Here's how the part is built. I have some questions about the finished solid (model axes, mm). Face numbers are marked on the shaded views. A direction names the side the tool comes from. Give positions to 0.01 mm unless a question says otherwise; leave off trailing zeros. Write each loop counter-clockwise with the first axis right and the second up, starting at its lowest first coordinate (ties: lowest second). Pieces come first, ordered by that corner, then holes. Notation, with made-up numbers: (84, 65) -> (107, 65) arc R12 ccw to (107, 88) -> close; hole circle Ø7 at (61, 83). An arc over 180 degrees is marked (long way). Put each result on its own line as item: value. Start each with the question number.
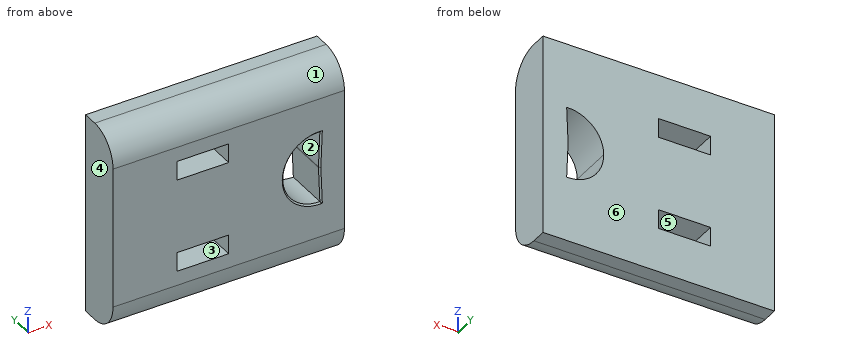
from build123d import *

# Parameters (mm, degrees)
F0_W         = 39.0713959932
F0_H         = 34.1874808073
F0_W_2       = 8.7503567338
F0_H_2       = 3.2559484243
F1_DEPTH     = 7.62
F2_R         = 5.08
F3_R         = 5.08
F4_T2_ANGLE  = 99.0884829953
F4_T4_ANGLE  = 99.0884829953
F4_T8_DEPTH  = 7.3218336241
F4_S9_R      = 6.0154186662
F4_T10_DEPTH = 5
F4_T14_DEPTH = 7.3218336241
F4_S15_R     = 6.0154186662
F4_T16_DEPTH = 5
F4_T21_DEPTH = 7.3218336241
F4_S22_R     = 6.0154186662
F4_T23_DEPTH = 5
F4_T26_ANGLE = 105.3128275547
F4_T33_ANGLE = 105.3128275547
F4_T37_DEPTH = 7.3218336241
F4_S38_R     = 6.0154186662
F4_T39_DEPTH = 5


# Not quite as in the source:
# - a fillet or chamfer that OpenCascade refuses, or shapes differently, is made with other operations: its cross-section is extruded or revolved along the edge and cut away or added


with BuildPart() as f1:
    # F0 (on Front) → F1 (new body)
    with BuildSketch(Plane.XZ):
        with Locations((19.5356979966, 17.0937404037)):
            Rectangle(F0_W, F0_H)
        with Locations((15.1605196297, 9.1573596001)):
            Rectangle(F0_W_2, F0_H_2, mode=Mode.SUBTRACT)
        with Locations((15.1605196297, 25.0301212072)):
            Rectangle(F0_W_2, F0_H_2, mode=Mode.SUBTRACT)
        with BuildLine():
            ThreePointArc((28.8283239088, 17.0937404037), (30.6523842077, 21.4714728973), (35.0814722478, 23.1670308858))
            Line((35.0814722478, 23.1670308858), (34.8434170056, 17.1563244854))
            Line((34.8434170056, 17.1563244854), (34.8434170056, 17.0311563219))
            Line((34.8434170056, 17.0311563219), (35.0814722478, 11.0204499215))
            ThreePointArc((35.0814722478, 11.0204499215), (30.6523842077, 12.71600791), (28.8283239088, 17.0937404037))
        make_face(mode=Mode.SUBTRACT)
    extrude(amount=F1_DEPTH)

    # F2
    f2_edges = [f1.edges().sort_by_distance(p)[0] for p in [
        (19.535698, -7.62, 34.187481),
    ]]
    fillet(f2_edges, radius=F2_R)

    # F3
    f3_edges = [f1.edges().sort_by_distance(p)[0] for p in [
        (19.535698, -7.62, 0),
    ]]
    fillet(f3_edges, radius=F3_R)

    # F4: chamfer of 0.254 on 4 edges, made by hand

    # F4_s1 → F4_t2 (revolve, cut)
    with BuildSketch(Plane(origin=(35.4623142005, 0, 1.4044921235), x_dir=(0, 1, 0), z_dir=(0.9992166354, 0, 0.0395741769))):
        Polygon((-7.62, 9.3694965041), (-7.366, 9.6234965041), (-7.62, 9.6234965041), align=None)
    revolve(axis=Axis((34.8434170056, -7.62, 17.0311563219), (0, 1, 0)), revolution_arc=F4_T2_ANGLE, mode=Mode.SUBTRACT)

    # F4_s3 → F4_t4 (revolve, cut)
    with BuildSketch(Plane(origin=(-1.5316236266, 0, 12.8056905764), x_dir=(0, 1, 0), z_dir=(0.1187584985, 0, -0.9929231688))):
        Polygon((-7.62, 30.3648766921), (-7.366, 30.6188766921), (-7.62, 30.6188766921), align=None)
    revolve(axis=Axis((34.8434170056, -7.62, 17.1563244854), (0, 1, 0)), revolution_arc=F4_T4_ANGLE, mode=Mode.SUBTRACT)


with BuildPart() as f4_tool6:
    # F4_s7 → F4_t8 (new body)
    with BuildSketch(Plane(origin=(0.9968897612, 0, 25.170677246), x_dir=(0, 1, 0), z_dir=(-0.0395741769, 0, -0.9992166354))):
        Polygon((-7.62, 34.3911744878), (-7.366, 34.1371744878), (-7.62, 34.1371744878), align=None)
    extrude(amount=F4_T8_DEPTH)

    # F4_s9 → F4_t10 (intersect, symmetric)
    with BuildSketch(Plane.XZ.offset(7.5)):
        with Locations((34.8434170056, 17.1563244854)):
            Circle(F4_S9_R)
    extrude(amount=F4_T10_DEPTH, both=True, mode=Mode.INTERSECT)


with BuildPart() as f1_1:
    add(f1.part)

    # F4_t5: cut F4_tool6
    add(f4_tool6.part, mode=Mode.SUBTRACT)


with BuildPart() as f4_tool12:
    # F4_s13 → F4_t14 (new body)
    with BuildSketch(Plane(origin=(-0.6447473432, 0, 16.2793599777), x_dir=(0, 1, 0), z_dir=(0.0395741769, 0, -0.9992166354))):
        Polygon((-7.62, 35.7441158998), (-7.366, 35.4901158998), (-7.62, 35.4901158998), align=None)
    extrude(amount=F4_T14_DEPTH)

    # F4_s15 → F4_t16 (intersect, symmetric)
    with BuildSketch(Plane.XZ.offset(7.5)):
        with Locations((34.8434170056, 17.0311563219)):
            Circle(F4_S15_R)
    extrude(amount=F4_T16_DEPTH, both=True, mode=Mode.INTERSECT)


with BuildPart() as f1_2:
    add(f1_1.part)

    # F4_t11: cut F4_tool12
    add(f4_tool12.part, mode=Mode.SUBTRACT)


with BuildPart() as f4_tool19:
    # F4_s20 → F4_t21 (new body)
    with BuildSketch(Plane(origin=(-0.6447473432, 0, 16.2793599777), x_dir=(0, 1, 0), z_dir=(0.0395741769, 0, -0.9992166354))):
        Polygon((-7.62, 35.7441158998), (-7.366, 35.4901158998), (-7.62, 35.4901158998), align=None)
    extrude(amount=F4_T21_DEPTH)

    # F4_s22 → F4_t23 (cut, symmetric)
    with BuildSketch(Plane.XZ.offset(7.5)):
        with Locations((34.8434170056, 17.0311563219)):
            Circle(F4_S22_R)
    extrude(amount=F4_T23_DEPTH, both=True, mode=Mode.SUBTRACT)


with BuildPart() as f4_tool24:
    # F4_s25 → F4_t26 (revolve)
    with BuildSketch(Plane(origin=(36.5710723448, 0, 5.4606046716), x_dir=(0, 1, 0), z_dir=(0.9890355378, 0, 0.1476777062))):
        Polygon((-7.62, 5.4294042858), (-7.366, 5.6834042858), (-7.62, 5.6834042858), align=None)
    revolve(axis=Axis((34.8434170056, -7.62, 17.0311563219), (0, 1, 0)), revolution_arc=F4_T26_ANGLE)

    split(bisect_by=Plane(origin=(35.4623142005, 0, 1.4044921235), x_dir=(0, 1, 0), z_dir=(0.9992166354, 0, 0.0395741769)), keep=Keep.TOP)


with BuildPart() as f4_tool19_1:
    add(f4_tool19.part)

    # F4_t28: intersect F4_tool24
    add(f4_tool24.part, mode=Mode.INTERSECT)


with BuildPart() as f1_3:
    add(f1_2.part)

    # F4_t17: cut F4_tool19
    add(f4_tool19_1.part, mode=Mode.SUBTRACT)


with BuildPart() as f4_tool31:
    # F4_s32 → F4_t33 (revolve)
    with BuildSketch(Plane(origin=(-1.5316236266, 0, 12.8056905764), x_dir=(0, 1, 0), z_dir=(0.1187584985, 0, -0.9929231688))):
        Polygon((-7.62, 30.3648766921), (-7.366, 30.6188766921), (-7.62, 30.6188766921), align=None)
    revolve(axis=Axis((34.8434170056, -7.62, 17.1563244854), (0, 1, 0)), revolution_arc=F4_T33_ANGLE)

    split(bisect_by=Plane(origin=(34.1104326349, 0, -1.3509505808), x_dir=(0, 1, 0), z_dir=(0.9992166354, 0, -0.0395741769)), keep=Keep.TOP)


with BuildPart() as f4_tool35:
    # F4_s36 → F4_t37 (new body)
    with BuildSketch(Plane(origin=(0.9968897612, 0, 25.170677246), x_dir=(0, 1, 0), z_dir=(-0.0395741769, 0, -0.9992166354))):
        Polygon((-7.62, 34.3911744878), (-7.366, 34.1371744878), (-7.62, 34.1371744878), align=None)
    extrude(amount=F4_T37_DEPTH)

    # F4_s38 → F4_t39 (cut, symmetric)
    with BuildSketch(Plane.XZ.offset(7.5)):
        with Locations((34.8434170056, 17.1563244854)):
            Circle(F4_S38_R)
    extrude(amount=F4_T39_DEPTH, both=True, mode=Mode.SUBTRACT)


with BuildPart() as f4_tool31_1:
    add(f4_tool31.part)

    # F4_t40: intersect F4_tool35
    add(f4_tool35.part, mode=Mode.INTERSECT)


with BuildPart() as f1_4:
    add(f1_3.part)

    # F4_t29: cut F4_tool31
    add(f4_tool31_1.part, mode=Mode.SUBTRACT)


solid = f1_4.part
1) I want a section at B-B, the plane z = 8. Write out the boundary of the cut face in (x, y), and give its area (3 significant figures).
2) I want a section at C-C, the plane y = -5. Write out the boundary of the cut face in (x, z).
3) Which directions (+Z, -Z, +X, -X, +Y, -Y) give clear straight access to the entire face, cutting with the end or side of a thin tool? Please do the marked faces 5 and 6.
4) I want a section at D-D, the plane x = 6.5. Write out the boundary of the cut face in (y, z), and give its area (3 significant figures).
5) I'm going to push flat-ended pins straight in: pin 1 Ø4 at (x, y) = (13.5, -5.5) entering from -Z; pin 2 Ø2.5 at (x, y) = (16, -5.5) entering from -Z; pin 3 Ø4 at (x, y) = (13, -5.5) entering from +Z. Where does each tip first touch, or does it pass through?
6) I need wall thicknesses on probe 1 along Z at (x, y) = (15, -2); probe 2 along X at (y, z) = (-5.5, 9); probe 3 along Z at (x, y) = (17, -6.75). Which ranges of each line are inside material? Lowest first, please.
7) Thinking about a two-plate mould opening in X: for the marked faces 1, 2, 3 and 4, which applies, released by +X, released by -X, zero draft, split by the parting line, or undercut?
8) I want a section at A-A, the plane x = 14.5. Write out the boundary of the cut face in (y, z), and give its area (3 significant figures).
Established:
1. outline: (0, -7.62) -> (10.79, -7.62) -> (10.79, 0) -> (0, 0) -> close; (19.54, -7.62) -> (39.07, -7.62) -> (39.07, 0) -> (19.54, 0) -> close
1. area: 231 mm2
2. outline: (0, 0.64) -> (39.07, 0.64) -> (39.07, 33.55) -> (0, 33.55) -> close; hole (10.79, 7.53) -> (19.54, 7.53) -> (19.54, 10.79) -> (10.79, 10.79) -> close; hole (10.79, 23.4) -> (19.54, 23.4) -> (19.54, 26.66) -> (10.79, 26.66) -> close; hole (28.83, 17.09) arc R6.02 ccw to (35.08, 11.02) -> (34.84, 17.03) -> (34.84, 17.16) -> (35.08, 23.17) arc R6.02 ccw to start
3. face 5: +Y, -Y
3. face 6: +Z, -Z, +X, -X, +Y
4. outline: (-7.62, 5.08) arc R5.08 ccw to (-2.54, 0) -> (0, 0) -> (0, 34.19) -> (-2.54, 34.19) arc R5.08 ccw to (-7.62, 29.11) -> close
4. area: 249 mm2
5. pin 1: stops at z = 0.09
5. pin 2: stops at z = 0.3
5. pin 3: stops at z = 34.1
6. probe 1: z = 0 to 7.53, 10.79 to 23.4, 26.66 to 34.19
6. probe 2: x = 0 to 10.79, 19.54 to 39.07
6. probe 3: z = 2.24 to 7.53, 10.79 to 23.4, 26.66 to 31.95
7. face 1: zero draft
7. face 2: undercut
7. face 3: undercut
7. face 4: released by -X
8. outline: (-7.62, 5.08) arc R5.08 ccw to (-2.54, 0) -> (0, 0) -> (0, 7.53) -> (-7.62, 7.53) -> close; (-7.62, 10.79) -> (0, 10.79) -> (0, 23.4) -> (-7.62, 23.4) -> close; (-7.62, 26.66) -> (0, 26.66) -> (0, 34.19) -> (-2.54, 34.19) arc R5.08 ccw to (-7.62, 29.11) -> close
8. area: 200 mm2
